Build history of the part. All positions in model axes, mm. A direction names the side the tool comes from. Give positions to 0.01 mm unless a question says otherwise; leave off trailing zeros. Loops run counter-clockwise (first coordinate to the right, second up) from the corner with the lowest first, then second, coordinate; pieces in that order, holes last.
1) Two-plate mould, pull along X, no slides. Class faces 1 (the flat face through (138, 37.998, 2)), 2 (the flat face through (139.7, 19, 1)), 3 (the flat face through (113, 88.9, 2)): +X half, -X half, draft (parallel to the pull), parting line (faces both ways), or undercut.
2) Wall check: line 1 (X direction, y = 4.5, z = 2.2); line 2 (X direction, y = 51.5, z = 1.7); line 3 (Y direction, x = 41, z = 1.7). Give the ranges that are in metal, low to high.
3) Band-saw the part on B-B on z = 2.1. List the corners of the cut face in (x, y), then the cut area to 3 significant figures.
4) Band-saw the part on C-C on y = 47.5. List the corners of the cut face in (x, z), then the cut area to 3 significant figures.
5) Band-saw the part on D-D on x = 62.5. List the corners of the cut face in (y, z).
6) 3-axis set-ups, long thin cutter, end or side, ignore diameter. For faces 4 (the flat face through (136.7, 32, 2)), 5 (the flat face through (55, 25.4, 2)), 6 (the flat face through (136.7, 6, 2)): which of +Z, -Z, +X, -X, +Y, -Y reach the whole face in a straight line?
7) Flat gauge pins, fed straight in: P1, Ø0.9, axis at x = 44.5, z = 1.5, coming from the -Y side; P2, Ø1.5, axis at x = 118, z = 1.5, coming from the -Y side; P3, Ø1.5, axis at x = 139, z = 1, coming from the -Y side. Where does each tip first touch, or does it go through?
8) Band-saw the part on A-A on y = 33. List the corners of the cut face in (x, z).
Autodesk Inventor part; units mm, degrees
ref_plane "YZ Plane" through (0, 0, 0) normal (1, 0, 0) x (0, 1, 0)
ref_plane "XZ Plane" through (0, 0, 0) normal (0, 1, 0) x (-1, 0, 0)
ref_plane "XY Plane" through (0, 0, 0) normal (0, 0, 1) x (1, 0, 0)
sketch "Sketch1" plane through (0, 0, 0) normal (0, 0, 1) x (1, 0, 0)
  line L0 (0, 0) -> (139.7, 0)
  line L1 (139.7, 0) -> (139.7, 101.6)
  line L2 (139.7, 101.6) -> (0, 101.6)
  line L3 (0, 101.6) -> (0, 0)
  dimension "d0" = 139.7
  dimension "d1" = 101.6
extrude "Extrusion1" add sketch "Sketch1" along normal blind 3
sketch "Sketch2" plane through (0, 0, 3) normal (0, 0, 1) x (1, 0, 0)
  line L0 (0, 0) -> (139.7, 0)
  line L1 (92.71, 0) -> (133.35, 0)
  line L2 (133.35, 0) -> (133.35, 88.9)
  line L3 (133.35, 88.9) -> (92.71, 88.9)
  line L4 (92.71, 88.9) -> (92.71, 0)
  line L5 (139.7, 0) -> (139.7, 101.6)
  dimension "d4" = 88.9
  dimension "d5" = 6.35
  dimension "d6" = 40.64
extrude "Extrusion2" cut sketch "Sketch2" against normal blind 3.5
sketch "Sketch3" plane through (0, 0, 3) normal (0, 0, 1) x (1, 0, 0)
  line L0 (15.24, 0) -> (92.71, 0)
  line L1 (92.71, 0) -> (92.71, 25.4)
  line L2 (92.71, 25.4) -> (15.24, 25.4)
  line L3 (15.24, 25.4) -> (15.24, 0)
  line L4 (133.35, 88.9) -> (133.35, 0)
  line L5 (133.35, 0) -> (139.7, 0)
  line L6 (139.7, 0) -> (139.7, 101.6)
  line L7 (139.7, 101.6) -> (0, 101.6)
  line L8 (0, 101.6) -> (0, 0)
  line L9 (0, 0) -> (92.71, 0)
  line L10 (92.71, 0) -> (92.71, 88.9)
  line L11 (92.71, 88.9) -> (133.35, 88.9)
  dimension "d9" = 25.4
  dimension "d10" = 0
  dimension "d12" = 0
  dimension "d15" = 15.24
extrude "Extrusion3" cut sketch "Sketch3" against normal blind 3.5 contours L3 L2 L1 L0
sketch "Sketch5" plane through (0, 0, 3) normal (0, 0, 1) x (1, 0, 0)
  line L0 (15.24, 0) -> (15.24, 25.4)
  line L1 (15.24, 25.4) -> (92.71, 25.4)
  line L2 (92.71, 25.4) -> (92.71, 88.9)
  line L3 (92.71, 88.9) -> (133.35, 88.9)
  line L4 (133.35, 88.9) -> (133.35, 0)
  line L5 (133.35, 0) -> (139.7, 0)
  line L6 (139.7, 0) -> (139.7, 101.6)
  line L7 (139.7, 101.6) -> (0, 101.6)
  line L8 (0, 101.6) -> (0, 0)
  line L9 (0, 0) -> (15.24, 0)
  line L10 (139.7, 0) -> (136.7, 0)
  line L11 (136.7, 0) -> (136.7, 12.5984)
  line L12 (136.7, 12.5984) -> (139.7, 12.5984)
  line L13 (139.7, 12.5984) -> (139.7, 0)
  line L14 (136.7, 25.4) -> (136.7, 37.9984)
  line L15 (136.7, 37.9984) -> (139.7, 37.9984)
  line L16 (139.7, 25.4) -> (136.7, 25.4)
  line L17 (139.7, 37.9984) -> (139.7, 25.4)
  line L18 (136.7, 50.8) -> (136.7, 63.3984)
  line L19 (136.7, 63.3984) -> (139.7, 63.3984)
  line L20 (139.7, 50.8) -> (136.7, 50.8)
  line L21 (139.7, 63.3984) -> (139.7, 50.8)
  line L22 (136.7, 76.2) -> (136.7, 88.7984)
  line L23 (136.7, 88.7984) -> (139.7, 88.7984)
  line L24 (139.7, 76.2) -> (136.7, 76.2)
  line L25 (139.7, 88.7984) -> (139.7, 76.2)
  line L26 (136.7, 101.6) -> (136.7, 114.1984)
  line L27 (136.7, 114.1984) -> (139.7, 114.1984)
  line L28 (139.7, 101.6) -> (136.7, 101.6)
  line L29 (139.7, 114.1984) -> (139.7, 101.6)
  dimension "d27" = 3
  dimension "d28" = 12.5984
  dimension "d31" = 25.4
extrude "Extrusion5" cut sketch "Sketch5" against normal blind 3 contours L26 L27 L29 L7 | L6 L24 L22 L23 | L11 L12 L6 L5 | L6 L20 L18 L19 | L16 L14 L15 L6
properties part number "CANIMDWall"
Findings below:
1. face 1: draft
1. face 2: +X half
1. face 3: undercut
2. line 1: x = 0 to 15.24, 133.35 to 136.7
2. line 2: x = 0 to 92.71, 133.35 to 136.7
2. line 3: y = 25.4 to 101.6
3. outline: (0, 0) - (15.24, 0) - (15.24, 25.4) - (92.71, 25.4) - (92.71, 88.9) - (133.35, 88.9) - (133.35, 0) - (136.7, 0) - (136.7, 12.6) - (139.7, 12.6) - (139.7, 25.4) - (136.7, 25.4) - (136.7, 38) - (139.7, 38) - (139.7, 50.8) - (136.7, 50.8) - (136.7, 63.4) - (139.7, 63.4) - (139.7, 76.2) - (136.7, 76.2) - (136.7, 88.8) - (139.7, 88.8) - (139.7, 101.6) - (0, 101.6) - close
3. area: 8,460 mm2
4. outline: (0, 0) - (92.71, 0) - (92.71, 3) - (0, 3) - close; (133.35, 0) - (139.7, 0) - (139.7, 3) - (133.35, 3) - close
4. area: 297 mm2
5. outline: (25.4, 0) - (101.6, 0) - (101.6, 3) - (25.4, 3) - close
6. face 4: +Z, -Z, +X
6. face 5: +Z, -Z, -Y
6. face 6: +Z, -Z, +X, -Y
7. P1: stops at y = 25.4
7. P2: stops at y = 88.9
7. P3: stops at y = 12.6
8. outline: (0, 0) - (92.71, 0) - (92.71, 3) - (0, 3) - close; (133.35, 0) - (136.7, 0) - (136.7, 3) - (133.35, 3) - close
